Verification items for the finished model (mm, model axes). Coordinates: 2 decimals unless noted, no trailing zeros. Write each loop counter-clockwise with the first axis right and the second up, starting at its lowest first coordinate (ties: lowest second). Pieces come first, ordered by that corner, then holes. Notation, with made-up numbers: (34, 40.5) -> (48, 40.5) arc R16 cw to (48, 54.5) -> close; hole circle Ø3 at (74, 58). An arc over 180 degrees is marked (long way). Answer in a Markdown table with one row per item.
```python
from build123d import *

# Parameters (mm, degrees)
ESQUISSE1_W             = 440
ESQUISSE1_H             = 220
BOSS_EXTRU_1_DEPTH      = 3
ESQUISSE2_R             = 5
ENL_V_MAT_EXTRU_1_DEPTH = 3
ESQUISSE3_W             = 5
ESQUISSE3_H             = 4
ENL_V_MAT_EXTRU_2_DEPTH = 3
ESQUISSE4_W             = 20
ESQUISSE4_H             = 3
ENL_V_MAT_EXTRU_3_DEPTH = 3
ESQUISSE5_W             = 3
ESQUISSE5_H             = 20
ENL_V_MAT_EXTRU_4_DEPTH = 3


with BuildPart() as part:
    # Esquisse1 → Boss.-Extru.1 (new body)
    with BuildSketch(Plane.XY):
        Rectangle(ESQUISSE1_W, ESQUISSE1_H)
    extrude(amount=BOSS_EXTRU_1_DEPTH)

    # Esquisse2 → Enlèv. mat.-Extru.1 (cut)
    with BuildSketch(Plane.XY.offset(3)):
        with Locations((0, -10)):
            Circle(ESQUISSE2_R)
    extrude(amount=-ENL_V_MAT_EXTRU_1_DEPTH, mode=Mode.SUBTRACT)

    # Esquisse3 → Enlèv. mat.-Extru.2 (cut)
    with BuildSketch(Plane.XY.offset(3)):
        with Locations((-201.5, 95)):
            Rectangle(ESQUISSE3_W, ESQUISSE3_H)
        with Locations((-168.5, 95)):
            Rectangle(ESQUISSE3_W, ESQUISSE3_H)
        with Locations((-168.5, 61)):
            Rectangle(ESQUISSE3_W, ESQUISSE3_H)
        with Locations((-201.5, 61)):
            Rectangle(ESQUISSE3_W, ESQUISSE3_H)
        with Locations((168.5, 61)):
            Rectangle(ESQUISSE3_W, ESQUISSE3_H)
        with Locations((201.5, 61)):
            Rectangle(ESQUISSE3_W, ESQUISSE3_H)
        with Locations((168.5, 95)):
            Rectangle(ESQUISSE3_W, ESQUISSE3_H)
        with Locations((201.5, 95)):
            Rectangle(ESQUISSE3_W, ESQUISSE3_H)
        with Locations((-16.5, -48)):
            Rectangle(ESQUISSE3_W, ESQUISSE3_H)
        with Locations((16.5, -48)):
            Rectangle(ESQUISSE3_W, ESQUISSE3_H)
        with Locations((16.5, -82)):
            Rectangle(ESQUISSE3_W, ESQUISSE3_H)
        with Locations((-16.5, -82)):
            Rectangle(ESQUISSE3_W, ESQUISSE3_H)
    extrude(amount=-ENL_V_MAT_EXTRU_2_DEPTH, mode=Mode.SUBTRACT)

    # Esquisse4 → Enlèv. mat.-Extru.3 (cut)
    with BuildSketch(Plane.XY.offset(3)):
        with Locations((-195, 105.5)):
            Rectangle(ESQUISSE4_W, ESQUISSE4_H)
        with Locations((-165, 105.5)):
            Rectangle(ESQUISSE4_W, ESQUISSE4_H)
        with Locations((-135, 105.5)):
            Rectangle(ESQUISSE4_W, ESQUISSE4_H)
        with Locations((-105, 105.5)):
            Rectangle(ESQUISSE4_W, ESQUISSE4_H)
        with Locations((-75, 105.5)):
            Rectangle(ESQUISSE4_W, ESQUISSE4_H)
        with Locations((-45, 105.5)):
            Rectangle(ESQUISSE4_W, ESQUISSE4_H)
        with Locations((-15, 105.5)):
            Rectangle(ESQUISSE4_W, ESQUISSE4_H)
        with Locations((15, 105.5)):
            Rectangle(ESQUISSE4_W, ESQUISSE4_H)
        with Locations((45, 105.5)):
            Rectangle(ESQUISSE4_W, ESQUISSE4_H)
        with Locations((75, 105.5)):
            Rectangle(ESQUISSE4_W, ESQUISSE4_H)
        with Locations((105, 105.5)):
            Rectangle(ESQUISSE4_W, ESQUISSE4_H)
        with Locations((135, 105.5)):
            Rectangle(ESQUISSE4_W, ESQUISSE4_H)
        with Locations((165, 105.5)):
            Rectangle(ESQUISSE4_W, ESQUISSE4_H)
        with Locations((195, 105.5)):
            Rectangle(ESQUISSE4_W, ESQUISSE4_H)
        with Locations((195, -105.5)):
            Rectangle(ESQUISSE4_W, ESQUISSE4_H)
        with Locations((165, -105.5)):
            Rectangle(ESQUISSE4_W, ESQUISSE4_H)
        with Locations((135, -105.5)):
            Rectangle(ESQUISSE4_W, ESQUISSE4_H)
        with Locations((105, -105.5)):
            Rectangle(ESQUISSE4_W, ESQUISSE4_H)
        with Locations((75, -105.5)):
            Rectangle(ESQUISSE4_W, ESQUISSE4_H)
        with Locations((45, -105.5)):
            Rectangle(ESQUISSE4_W, ESQUISSE4_H)
        with Locations((15, -105.5)):
            Rectangle(ESQUISSE4_W, ESQUISSE4_H)
        with Locations((-15, -105.5)):
            Rectangle(ESQUISSE4_W, ESQUISSE4_H)
        with Locations((-45, -105.5)):
            Rectangle(ESQUISSE4_W, ESQUISSE4_H)
        with Locations((-75, -105.5)):
            Rectangle(ESQUISSE4_W, ESQUISSE4_H)
        with Locations((-105, -105.5)):
            Rectangle(ESQUISSE4_W, ESQUISSE4_H)
        with Locations((-135, -105.5)):
            Rectangle(ESQUISSE4_W, ESQUISSE4_H)
        with Locations((-165, -105.5)):
            Rectangle(ESQUISSE4_W, ESQUISSE4_H)
        with Locations((-195, -105.5)):
            Rectangle(ESQUISSE4_W, ESQUISSE4_H)
    extrude(amount=-ENL_V_MAT_EXTRU_3_DEPTH, mode=Mode.SUBTRACT)

    # Esquisse5 → Enlèv. mat.-Extru.4 (cut)
    with BuildSketch(Plane.XY.offset(3)):
        with Locations((-215.5, -90)):
            Rectangle(ESQUISSE5_W, ESQUISSE5_H)
        with Locations((-215.5, -60)):
            Rectangle(ESQUISSE5_W, ESQUISSE5_H)
        with Locations((-215.5, -30)):
            Rectangle(ESQUISSE5_W, ESQUISSE5_H)
        with Locations((-215.5, 0)):
            Rectangle(ESQUISSE5_W, ESQUISSE5_H)
        with Locations((-215.5, 30)):
            Rectangle(ESQUISSE5_W, ESQUISSE5_H)
        with Locations((-215.5, 60)):
            Rectangle(ESQUISSE5_W, ESQUISSE5_H)
        with Locations((-215.5, 90)):
            Rectangle(ESQUISSE5_W, ESQUISSE5_H)
        with Locations((215.5, 90)):
            Rectangle(ESQUISSE5_W, ESQUISSE5_H)
        with Locations((215.5, 60)):
            Rectangle(ESQUISSE5_W, ESQUISSE5_H)
        with Locations((215.5, 30)):
            Rectangle(ESQUISSE5_W, ESQUISSE5_H)
        with Locations((215.5, 0)):
            Rectangle(ESQUISSE5_W, ESQUISSE5_H)
        with Locations((215.5, -30)):
            Rectangle(ESQUISSE5_W, ESQUISSE5_H)
        with Locations((215.5, -60)):
            Rectangle(ESQUISSE5_W, ESQUISSE5_H)
        with Locations((215.5, -90)):
            Rectangle(ESQUISSE5_W, ESQUISSE5_H)
    extrude(amount=-ENL_V_MAT_EXTRU_4_DEPTH, mode=Mode.SUBTRACT)


solid = part.part
```
1. Thickness scan on line 1 (X direction, y = -97, z = 0.8); line 2 (Y direction, x = 197.5, z = 1.5); line 3 (Y direction, x = 0, z = 0.75). Record the ranges inside material, lowest first. Write a range as from..to.
Geometry says:
| item | result |
|---|---|
| line 1 | -220..-217, -214..214, 217..220 |
| line 2 | -110..-107, -104..104, 107..110 |
| line 3 | -110..-15, -5..110 |
2. Section check B-B, the plane x = -159. Record the boundary of the cut face in (y, z).
Geometry says:
| item | result |
|---|---|
| outline | (-110, 0) -> (-107, 0) -> (-107, 3) -> (-110, 3) -> close; (-104, 0) -> (104, 0) -> (104, 3) -> (-104, 3) -> close; (107, 0) -> (110, 0) -> (110, 3) -> (107, 3) -> close |
3. Section check C-C, the plane z = 2.15. State how many separate pieces and enclosed holes the cut face has, plus the area to 3 significant figures.
Geometry says:
| item | result |
|---|---|
| separate pieces | 1 |
| enclosed holes | 55 |
| area | 94,000 mm^2 |
4. Section check A-A, the plane x = 0. Record the boundary of the cut face in (y, z).
Geometry says:
| item | result |
|---|---|
| outline | (-110, 0) -> (-15, 0) -> (-15, 3) -> (-110, 3) -> close; (-5, 0) -> (110, 0) -> (110, 3) -> (-5, 3) -> close |
5. Mould release check, pull along X, two halves, no side actions. Record for faces 1 (the cylindrical face through (-0.651, -5.043, 1.521)), 2 (the flat face through (-3, 2, 0)): released by +X, released by -X, zero draft, split by the parting line, or undercut.
Geometry says:
| item | result |
|---|---|
| face 1 | undercut |
| face 2 | zero draft |
